```python
from build123d import *

# Parameters (mm, degrees)
SKETCH1_W               = 100
SKETCH1_H               = 100
BOSS_EXTRUDE1_DEPTH     = 3
SKETCH2_R               = 1.75
CUT_EXTRUDE1_DEPTH      = 71.774289117
MIRROR2_COPY_1_SKETCH_R = 1.75
MIRROR2_COPY_1_DEPTH    = 71.774289117
CHAMFER1_SIZE           = 5
SKETCH9_R               = 1.75
BOSS_EXTRUDE2_DEPTH     = 3
CUT_EXTRUDE4_REACH      = 92.189
SKETCH6_R               = 1.75
SKETCH10_R              = 2.15
SKETCH10_R_2            = 1.75
SKETCH10_R_3            = 1.9
SKETCH10_R_4            = 1.5
CUT_EXTRUDE5_DEPTH      = 3
SKETCH13_R              = 1.75
CUT_EXTRUDE6_DEPTH      = 3


with BuildPart() as part:
    # Sketch1 → Boss-Extrude1 (new body)
    with BuildSketch(Plane(origin=(0, 0, 0), x_dir=(1, 0, 0), z_dir=(0, 1, 0))):
        Rectangle(SKETCH1_W, SKETCH1_H)
    extrude(amount=BOSS_EXTRUDE1_DEPTH)

    # Sketch2 → Cut-Extrude1 (cut, through all)
    with BuildSketch(Plane(origin=(0, 3, 0), x_dir=(1, 0, 0), z_dir=(0, 1, 0))):
        with Locations(Location((-40, 43, 0), (0, 0, 270))):
            Circle(SKETCH2_R)
    cut_extrude1 = extrude(amount=-CUT_EXTRUDE1_DEPTH, mode=Mode.SUBTRACT)

    # Mirror1: Cut-Extrude1 across plane
    add(cut_extrude1.mirror(Plane(origin=(0, 0, 0), x_dir=(0, 0, 1), z_dir=(1, 0, 0))), mode=Mode.SUBTRACT)

    # Mirror2: Cut-Extrude1 across plane
    add(cut_extrude1.mirror(Plane.XY), mode=Mode.SUBTRACT)

    # Mirror2 copy 1 sketch → Mirror2 copy 1 (cut, through all)
    with BuildSketch(Plane(origin=(0, 3, 0), x_dir=(-1, 0, 0), z_dir=(0, 1, 0))):
        with Locations(Location((-40, 43, 0), (0, 0, 270))):
            Circle(MIRROR2_COPY_1_SKETCH_R)
    extrude(amount=-MIRROR2_COPY_1_DEPTH, mode=Mode.SUBTRACT)

    # Chamfer1
    chamfer1_edges = [part.edges().sort_by_distance(p)[0] for p in [
        (-50, 1.5, -50),
        (50, 1.5, -50),
        (50, 1.5, 50),
        (-50, 1.5, 50),
    ]]
    chamfer(chamfer1_edges, length=CHAMFER1_SIZE)

    # Sketch9 → Boss-Extrude2 (add)
    with BuildSketch(Plane(origin=(0, 3, 0), x_dir=(1, 0, 0), z_dir=(0, 1, 0))):
        with BuildLine():
            Line((45, 50), (50, 45))
            Line((50, 45), (50, 55.901699437))
            ThreePointArc((50, 55.901699437), (0, 75), (-50, 55.901699437))
            Line((-50, 55.901699437), (-50, 45))
            Line((-50, 45), (-45, 50))
            Line((-45, 50), (45, 50))
        make_face()
        with Locations(Location((-30.5, 61.5, 0), (0, 0, 270))):
            Circle(SKETCH9_R, mode=Mode.SUBTRACT)
    extrude(amount=-BOSS_EXTRUDE2_DEPTH)

    # Sketch6 → Cut-Extrude4 (cut, up to next)
    with BuildSketch(Plane(origin=(0, 3, 0), x_dir=(1, 0, 0), z_dir=(0, 1, 0)), mode=Mode.PRIVATE) as cut_extrude4_sk1:
        with Locations(Location((-18.23, 10.76, 0), (0, 0, 270))):
            Circle(SKETCH6_R)
    cut_extrude4_tool1 = extrude(cut_extrude4_sk1.sketch, amount=-CUT_EXTRUDE4_REACH, mode=Mode.PRIVATE) & part.part
    # Sketch6 → Cut-Extrude4 (cut, up to next)
    with BuildSketch(Plane(origin=(0, 3, 0), x_dir=(1, 0, 0), z_dir=(0, 1, 0)), mode=Mode.PRIVATE) as cut_extrude4_sk2:
        with Locations(Location((-19.5, -37.5, 0), (0, 0, 270))):
            Circle(SKETCH6_R)
    cut_extrude4_tool2 = extrude(cut_extrude4_sk2.sketch, amount=-CUT_EXTRUDE4_REACH, mode=Mode.PRIVATE) & part.part
    # Sketch6 → Cut-Extrude4 (cut, up to next)
    with BuildSketch(Plane(origin=(0, 3, 0), x_dir=(1, 0, 0), z_dir=(0, 1, 0)), mode=Mode.PRIVATE) as cut_extrude4_sk3:
        with Locations(Location((32.57, -32.42, 0), (0, 0, 270))):
            Circle(SKETCH6_R)
    cut_extrude4_tool3 = extrude(cut_extrude4_sk3.sketch, amount=-CUT_EXTRUDE4_REACH, mode=Mode.PRIVATE) & part.part
    # Sketch6 → Cut-Extrude4 (cut, up to next)
    with BuildSketch(Plane(origin=(0, 3, 0), x_dir=(1, 0, 0), z_dir=(0, 1, 0)), mode=Mode.PRIVATE) as cut_extrude4_sk4:
        with Locations(Location((32.57, -4.48, 0), (0, 0, 270))):
            Circle(SKETCH6_R)
    cut_extrude4_tool4 = extrude(cut_extrude4_sk4.sketch, amount=-CUT_EXTRUDE4_REACH, mode=Mode.PRIVATE) & part.part
    add(cut_extrude4_tool1.solids().sort_by_distance((-18.23, 3, -10.76))[0], mode=Mode.SUBTRACT)
    add(cut_extrude4_tool2.solids().sort_by_distance((-19.5, 3, 37.5))[0], mode=Mode.SUBTRACT)
    add(cut_extrude4_tool3.solids().sort_by_distance((32.57, 3, 32.42))[0], mode=Mode.SUBTRACT)
    add(cut_extrude4_tool4.solids().sort_by_distance((32.57, 3, 4.48))[0], mode=Mode.SUBTRACT)

    # Sketch10 → Cut-Extrude5 (cut)
    # profile 1 of 26: a face of its own
    with BuildSketch(Plane(origin=(0, 3, 0), x_dir=(1, 0, 0), z_dir=(0, 1, 0))):
        with Locations(Location((-40, 43, 0), (0, 0, 270))):
            Circle(SKETCH10_R)
        with Locations((-40, 43)):
            Circle(SKETCH10_R_2, mode=Mode.SUBTRACT)
    # profile 2 of 26: a face of its own
    with BuildSketch(Plane(origin=(0, 3, 0), x_dir=(1, 0, 0), z_dir=(0, 1, 0))):
        with Locations((-40, 43)):
            Circle(SKETCH10_R_2)
    # profile 3 of 26: a face of its own
    with BuildSketch(Plane(origin=(0, 3, 0), x_dir=(1, 0, 0), z_dir=(0, 1, 0))):
        with Locations(Location((-30.5, 61.5, 0), (0, 0, 270))):
            Circle(SKETCH10_R_3)
        with Locations((-30.5, 61.5)):
            Circle(SKETCH10_R_2, mode=Mode.SUBTRACT)
    # profile 4 of 26: a face of its own
    with BuildSketch(Plane(origin=(0, 3, 0), x_dir=(1, 0, 0), z_dir=(0, 1, 0))):
        with Locations((-30.5, 61.5)):
            Circle(SKETCH10_R_2)
        with Locations((-30.5, 61.5)):
            Circle(SKETCH10_R_4, mode=Mode.SUBTRACT)
    # profile 5 of 26: a face of its own
    with BuildSketch(Plane(origin=(0, 3, 0), x_dir=(1, 0, 0), z_dir=(0, 1, 0))):
        with Locations((-30.5, 61.5)):
            Circle(SKETCH10_R_4)
    # profile 6 of 26: a face of its own
    with BuildSketch(Plane(origin=(0, 3, 0), x_dir=(1, 0, 0), z_dir=(0, 1, 0))):
        with Locations(Location((-30.5, 34.5, 0), (0, 0, 270))):
            Circle(SKETCH10_R_3)
        with Locations((-30.5, 34.5)):
            Circle(SKETCH10_R_4, mode=Mode.SUBTRACT)
    # profile 7 of 26: a face of its own
    with BuildSketch(Plane(origin=(0, 3, 0), x_dir=(1, 0, 0), z_dir=(0, 1, 0))):
        with Locations((-30.5, 34.5)):
            Circle(SKETCH10_R_4)
    # profile 8 of 26: a face of its own
    with BuildSketch(Plane(origin=(0, 3, 0), x_dir=(1, 0, 0), z_dir=(0, 1, 0))):
        with Locations(Location((-18.23, 10.76, 0), (0, 0, 270))):
            Circle(SKETCH10_R)
        with Locations((-18.23, 10.76)):
            Circle(SKETCH10_R_2, mode=Mode.SUBTRACT)
    # profile 9 of 26: a face of its own
    with BuildSketch(Plane(origin=(0, 3, 0), x_dir=(1, 0, 0), z_dir=(0, 1, 0))):
        with Locations((-18.23, 10.76)):
            Circle(SKETCH10_R_2)
    # profile 10 of 26: a face of its own
    with BuildSketch(Plane(origin=(0, 3, 0), x_dir=(1, 0, 0), z_dir=(0, 1, 0))):
        with Locations(Location((-19.5, -37.5, 0), (0, 0, 270))):
            Circle(SKETCH10_R)
        with Locations((-19.5, -37.5)):
            Circle(SKETCH10_R_2, mode=Mode.SUBTRACT)
    # profile 11 of 26: a face of its own
    with BuildSketch(Plane(origin=(0, 3, 0), x_dir=(1, 0, 0), z_dir=(0, 1, 0))):
        with Locations((-19.5, -37.5)):
            Circle(SKETCH10_R_2)
    # profile 12 of 26: a face of its own
    with BuildSketch(Plane(origin=(0, 3, 0), x_dir=(1, 0, 0), z_dir=(0, 1, 0))):
        with Locations(Location((-40, -43, 0), (0, 0, 270))):
            Circle(SKETCH10_R)
        with Locations((-40, -43)):
            Circle(SKETCH10_R_2, mode=Mode.SUBTRACT)
    # profile 13 of 26: a face of its own
    with BuildSketch(Plane(origin=(0, 3, 0), x_dir=(1, 0, 0), z_dir=(0, 1, 0))):
        with Locations((-40, -43)):
            Circle(SKETCH10_R_2)
    # profile 14 of 26: a face of its own
    with BuildSketch(Plane(origin=(0, 3, 0), x_dir=(1, 0, 0), z_dir=(0, 1, 0))):
        with Locations(Location((40, -43, 0), (0, 0, 270))):
            Circle(SKETCH10_R)
        with Locations((40, -43)):
            Circle(SKETCH10_R_2, mode=Mode.SUBTRACT)
    # profile 15 of 26: a face of its own
    with BuildSketch(Plane(origin=(0, 3, 0), x_dir=(1, 0, 0), z_dir=(0, 1, 0))):
        with Locations((40, -43)):
            Circle(SKETCH10_R_2)
    # profile 16 of 26: a face of its own
    with BuildSketch(Plane(origin=(0, 3, 0), x_dir=(1, 0, 0), z_dir=(0, 1, 0))):
        with Locations(Location((32.57, -32.42, 0), (0, 0, 270))):
            Circle(SKETCH10_R)
        with Locations((32.57, -32.42)):
            Circle(SKETCH10_R_2, mode=Mode.SUBTRACT)
    # profile 17 of 26: a face of its own
    with BuildSketch(Plane(origin=(0, 3, 0), x_dir=(1, 0, 0), z_dir=(0, 1, 0))):
        with Locations((32.57, -32.42)):
            Circle(SKETCH10_R_2)
    # profile 18 of 26: a face of its own
    with BuildSketch(Plane(origin=(0, 3, 0), x_dir=(1, 0, 0), z_dir=(0, 1, 0))):
        with Locations(Location((32.57, -4.48, 0), (0, 0, 270))):
            Circle(SKETCH10_R)
        with Locations((32.57, -4.48)):
            Circle(SKETCH10_R_2, mode=Mode.SUBTRACT)
    # profile 19 of 26: a face of its own
    with BuildSketch(Plane(origin=(0, 3, 0), x_dir=(1, 0, 0), z_dir=(0, 1, 0))):
        with Locations((32.57, -4.48)):
            Circle(SKETCH10_R_2)
    # profile 20 of 26: a face of its own
    with BuildSketch(Plane(origin=(0, 3, 0), x_dir=(1, 0, 0), z_dir=(0, 1, 0))):
        with Locations(Location((40, 43, 0), (0, 0, 270))):
            Circle(SKETCH10_R)
        with Locations((40, 43)):
            Circle(SKETCH10_R_2, mode=Mode.SUBTRACT)
    # profile 21 of 26: a face of its own
    with BuildSketch(Plane(origin=(0, 3, 0), x_dir=(1, 0, 0), z_dir=(0, 1, 0))):
        with Locations((40, 43)):
            Circle(SKETCH10_R_2)
    # profile 22 of 26: a face of its own
    with BuildSketch(Plane(origin=(0, 3, 0), x_dir=(1, 0, 0), z_dir=(0, 1, 0))):
        with Locations(Location((11.05, 34.5, 0), (0, 0, 270))):
            Circle(SKETCH10_R_3)
        with Locations((11.05, 34.5)):
            Circle(SKETCH10_R_4, mode=Mode.SUBTRACT)
    # profile 23 of 26: a face of its own
    with BuildSketch(Plane(origin=(0, 3, 0), x_dir=(1, 0, 0), z_dir=(0, 1, 0))):
        with Locations((11.05, 34.5)):
            Circle(SKETCH10_R_4)
    # profile 24 of 26: a face of its own
    with BuildSketch(Plane(origin=(0, 3, 0), x_dir=(1, 0, 0), z_dir=(0, 1, 0))):
        with Locations(Location((11.05, 61.5, 0), (0, 0, 270))):
            Circle(SKETCH10_R_3)
        with Locations((11.05, 61.5)):
            Circle(SKETCH10_R_2, mode=Mode.SUBTRACT)
    # profile 25 of 26: a face of its own
    with BuildSketch(Plane(origin=(0, 3, 0), x_dir=(1, 0, 0), z_dir=(0, 1, 0))):
        with Locations((11.05, 61.5)):
            Circle(SKETCH10_R_2)
        with Locations((11.05, 61.5)):
            Circle(SKETCH10_R_4, mode=Mode.SUBTRACT)
    # profile 26 of 26: a face of its own
    with BuildSketch(Plane(origin=(0, 3, 0), x_dir=(1, 0, 0), z_dir=(0, 1, 0))):
        with Locations((11.05, 61.5)):
            Circle(SKETCH10_R_4)
    extrude(amount=-CUT_EXTRUDE5_DEPTH, mode=Mode.SUBTRACT)

    # Sketch13 → Cut-Extrude6 (cut)
    with BuildSketch(Plane(origin=(0, 3, 0), x_dir=(1, 0, 0), z_dir=(0, 1, 0))):
        with Locations(Location((20.855220052, 45.129061124, 0), (0, 0, 270))):
            Circle(SKETCH13_R)
        with Locations(Location((20.834109359, 22.297361761, 0), (0, 0, 270))):
            Circle(SKETCH13_R)
    extrude(amount=-CUT_EXTRUDE6_DEPTH, mode=Mode.SUBTRACT)


solid = part.part
```
Part model, mm, in its own coordinate system. Round coordinates to 2 decimals unless told otherwise and drop trailing zeros. Write each loop counter-clockwise with the first axis right and the second up, starting at its lowest first coordinate (ties: lowest second). Pieces come first, ordered by that corner, then holes. Notation, with made-up numbers: M 17.5,42.25 L 21.5,42.25 A23 cw 21.5,65.25 Z; hole C -39.75,-34 d3. An arc over 180 degrees is marked long. Answer as CSV lines item,"result". Start each with the question number.
1) Mould opens along X. For faces 1 (the face through (-38.19, 1.52, -41.84)), 2 (the face through (-47, 1, 48)), 3 (the face through (-1, 0, -13)) say: +X half, -X half, draft (parallel to the pull), parting line (faces both ways), or undercut.
2) Band-saw the part on B-B (z = -61.5). List the corners of the cut face in (x, y), then the cut area to 3 significant figures.
3) Band-saw the part on A-A (z = 32.42). List the corners of the cut face in (x, y).
4) Drill centre lines: L1, parallel to X at y = 1.5, z = 43; L2, parallel to Z at x = 10.5, y = 1; L3, parallel to Z at x = -30, y = 0.3. Where is each one in solid material? Low to high.
5) Band-saw the part on D-D (y = 0.75). Count the separate pieces of the cut face and the enclosed holes in it, then the cut area to 3 significant figures.
6) Band-saw the part on C-C (x = -40). List the corners of the cut face in (y, z).
Worked out:
1,face 1,"undercut"
1,face 2,"-X half"
1,face 3,"draft"
2,outline,"M -42.93,0 L -32.4,0 L -32.4,3 L -42.93,3 Z; M -28.6,0 L 9.15,0 L 9.15,3 L -28.6,3 Z; M 12.95,0 L 42.93,0 L 42.93,3 L 12.95,3 Z"
2,area,"235 mm²"
3,outline,"M -50,0 L 30.42,0 L 30.42,3 L -50,3 Z; M 34.72,0 L 50,0 L 50,3 L 34.72,3 Z"
4,L1,"-50 to -42.15, -37.85 to 37.85, 42.15 to 50"
4,L2,"-74.26 to -63.32, -59.68 to -36.32, -32.68 to 50"
4,L3,"-68.74 to -63.33, -59.67 to -36.33, -32.67 to 50"
5,separate pieces,"1"
5,enclosed holes,"14"
5,area,"11,700 mm²"
6,outline,"M 0,-63.44 L 3,-63.44 L 3,-45.15 L 0,-45.15 Z; M 0,-40.85 L 3,-40.85 L 3,40.85 L 0,40.85 Z; M 0,45.15 L 3,45.15 L 3,50 L 0,50 Z"
